Check sheet for the modelled part. Datum: model origin and axes. Units: mm. Face numbers are marked on the shaded views. Round coordinates to 2 decimals unless told otherwise and drop trailing zeros. Write each loop counter-clockwise with the first axis right and the second up, starting at its lowest first coordinate (ties: lowest second). Pieces come first, ordered by that corner, then holes. Notation, with made-up numbers: M 35,86 L 64,86 A21 ccw 64,97 Z; hole C 45,64 d8. An arc over 180 degrees is marked long. Answer in a Markdown table with one row per item.
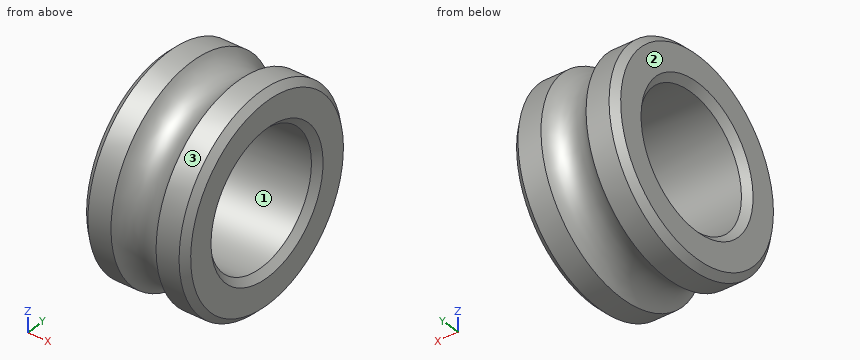
```python
from build123d import *

# Parameters (mm, degrees)
PAH1_SIZE = 0.5


with BuildPart() as part:
    # Çizim1 → Döndür1 (revolve)
    with BuildSketch(Plane.XY, mode=Mode.PRIVATE) as d_nd_r1_sk:
        with BuildLine():
            Line((-0.523961526, 5), (-8.523961526, 5))
            Line((-8.523961526, 5), (-8.523961526, 8))
            Line((-8.523961526, 8), (-6.256012333, 8))
            ThreePointArc((-6.256012333, 8), (-4.523961526, 7), (-2.791910718, 8))
            Line((-2.791910718, 8), (-0.523961526, 8))
            Line((-0.523961526, 8), (-0.523961526, 5))
        make_face()
    revolve(d_nd_r1_sk.sketch.rotate(Axis((0, 0, 0), (-1, 0, 0)), 90), axis=Axis((0, 0, 0), (-1, 0, 0)))

    # Pah1
    pah1_edges = [part.edges().sort_by_distance(p)[0] for p in [
        (-0.523961526, 0, 5),
        (-8.523961526, 0, 5),
        (-8.523961526, 0, 8),
        (-0.523961526, 0, 8),
    ]]
    chamfer(pah1_edges, length=PAH1_SIZE)


solid = part.part
```
1. Section check B-B, the plane x = -1.5. Record the cut outline in (y, z), and give its area (3 significant figures).
Found:
| item | result |
|---|---|
| outline | C 0,0 d16; hole C 0,0 d10 |
| area | 123 mm2 |
2. Scan lines: L1, parallel to Y at x = -2.5, z = 0; L2, parallel to Z at x = -3, y = -4.5; L3, parallel to Y at x = -6, z = 3. Record each from-to range of solid material in increasing order.
Found:
| item | result |
|---|---|
| L1 | y = -8 to -5, 5 to 8 |
| L2 | z = -6.25 to -2.18, 2.18 to 6.25 |
| L3 | y = -7.04 to -4, 4 to 7.04 |
3. Section check A-A, the plane z = 0. Record the cut outline in (x, y).
Found:
| item | result |
|---|---|
| outline | M -8.52,-7.5 L -8.02,-8 L -6.26,-8 A2 cw -2.79,-8 L -1.02,-8 L -0.52,-7.5 L -0.52,-5.5 L -1.02,-5 L -8.02,-5 L -8.52,-5.5 Z; M -8.52,5.5 L -8.02,5 L -1.02,5 L -0.52,5.5 L -0.52,7.5 L -1.02,8 L -2.79,8 A2 cw -6.26,8 L -8.02,8 L -8.52,7.5 Z |
4. Draft check along Z on the marked faces 1, 2 and 3. Enter one of: +Z half, -Z half, draft (parallel to the pull), parting line (faces both ways), or undercut.
Found:
| item | result |
|---|---|
| face 1 | undercut |
| face 2 | draft |
| face 3 | parting line |
5. Section check C-C, the plane x = -4. Record the cut outline in (y, z), and give its area (3 significant figures).
Found:
| item | result |
|---|---|
| outline | C 0,0 d14.14; hole C 0,0 d10 |
| area | 78.5 mm2 |
6. Go/stop test with flat-tipped pins: pin 1 (1 mm diameter, centred on x = -1.5, z = 3, fed in from +Y); pin 2 (6 mm diameter, centred on y = 0, z = 0, fed in from -X); pin 3 (1.5 mm diameter, centred on x = -4, y = 3.5, fed in from -Z). Record where each tip stops, or that it passes through.
Found:
| item | result |
|---|---|
| pin 1 | stops at y = 7.6 |
| pin 2 | passes through |
| pin 3 | stops at z = -6.69 |
